Here's how the part is built. I have some questions about the finished solid (model axes, mm). A direction names the side the tool comes from. Round coordinates to 2 decimals unless told otherwise and drop trailing zeros. Write each loop counter-clockwise with the first axis right and the second up, starting at its lowest first coordinate (ties: lowest second). Pieces come first, ordered by that corner, then holes. Notation, with made-up numbers: (66, -31) -> (105, -31) arc R28 cw to (105, -13) -> close; hole circle Ø11 at (81.5, 58.5). An arc over 180 degrees is marked (long way). Put each result on its own line as item: value. Start each with the question number.
1) Which directions (+Z, -Z, +X, -X, +Y, -Y) give clear straight access to the entire face, cutting with the end or side of a thin tool? Please do faces 1 (the flat face through (7.4, 14, 9)), 2 (the flat face through (7, 21, 0)).
2) I want a section at A-A, the plane x = 0. List the corners of the cut face in (y, z) for me, then the cut area to 3 significant figures.
3) I want a section at C-C, the plane z = 0. List the corners of the cut face in (x, y) for me.
4) Will these pins go through, and if not, where does the flat tip stop? P1, Ø6, axis at x = 2, z = -4.5, coming from the +Y side; P2, Ø6, axis at x = 6, y = 15.5, coming from the +Z side; P3, Ø3, axis at y = 8, z = -6, coming from the -X side; P4, Ø5, axis at y = 10, z = 0, coming from the -X side.
5) We'd pull the mould along Z, two halves only. Please class faces 3 (the flat face through (7.4, 14, -9)), 4 (the flat face through (-2.4, 0, 1.9)), 5 (the cylindrical face through (8.521, 32.727, 0.358)): released by +Z, released by -Z, zero draft, split by the parting line, or undercut.
6) I want a section at D-D, the plane z = 7. List the corners of the cut face in (x, y) for me.
7) I want a section at B-B, the plane y = 10. List the corners of the cut face in (x, z) for me.
8) If I drill on line 1 along Y through (x, z) = (8.2, 0); line 2 along Z through (x, y) = (0, 0.8); line 3 along X through (y, z) = (22, 4.5), over which ranges is the centre line in solid material (lowest first)? Write a range as [from, to].
from build123d import *

# Parameters (mm, degrees)
SKETCH_1_W          = 20
SKETCH_1_H          = 18
EXTRUDE_1_DEPTH     = 3
SKETCH_2_W          = 3
SKETCH_2_H          = 18
EXTRUDE_2_DEPTH     = 37
SKETCH_4_R          = 2.75
CUT_EXTRUDE_1_DEPTH = 41
SKETCH_5_R          = 2.75
CUT_EXTRUDE_2_DEPTH = 21


with BuildPart() as part:
    # 草图1 → 凸台-拉伸1 (new body)
    with BuildSketch(Plane(origin=(0, 0, 0), x_dir=(1, 0, 0), z_dir=(0, 1, 0))):
        Rectangle(SKETCH_1_W, SKETCH_1_H)
    extrude(amount=EXTRUDE_1_DEPTH)

    # 草图2 → 凸台-拉伸2 (add)
    with BuildSketch(Plane(origin=(0, 3, 0), x_dir=(1, 0, 0), z_dir=(0, 1, 0))):
        with Locations((8.5, 0)):
            Rectangle(SKETCH_2_W, SKETCH_2_H)
    extrude(amount=EXTRUDE_2_DEPTH)

    # 草图4 → 切除-拉伸1 (cut, through all)
    with BuildSketch(Plane.XZ):
        Circle(SKETCH_4_R)
    extrude(amount=-CUT_EXTRUDE_1_DEPTH, mode=Mode.SUBTRACT)

    # 草图5 → 切除-拉伸2 (cut, through all)
    with BuildSketch(Plane(origin=(10, 0, 0), x_dir=(0, 0, -1), z_dir=(1, 0, 0))):
        with Locations((0, 10)):
            Circle(SKETCH_5_R)
        with Locations((0, 30)):
            Circle(SKETCH_5_R)
    extrude(amount=-CUT_EXTRUDE_2_DEPTH, mode=Mode.SUBTRACT)


solid = part.part
Findings:
1. face 1: +Z, +X, -X, +Y, -Y
1. face 2: +Z, -Z, -X, +Y
2. outline: (0, -9) -> (3, -9) -> (3, -2.75) -> (0, -2.75) -> close; (0, 2.75) -> (3, 2.75) -> (3, 9) -> (0, 9) -> close
2. area: 37.5 mm2
3. outline: (-10, 0) -> (-2.75, 0) -> (-2.75, 3) -> (-10, 3) -> close; (2.75, 0) -> (10, 0) -> (10, 7.25) -> (7, 7.25) -> (7, 3) -> (2.75, 3) -> close; (7, 12.75) -> (10, 12.75) -> (10, 27.25) -> (7, 27.25) -> close; (7, 32.75) -> (10, 32.75) -> (10, 40) -> (7, 40) -> close
4. P1: stops at y = 3
4. P2: stops at z = 9
4. P3: stops at x = 7
4. P4: passes through
5. face 3: released by -Z
5. face 4: zero draft
5. face 5: undercut
6. outline: (-10, 0) -> (10, 0) -> (10, 40) -> (7, 40) -> (7, 3) -> (-10, 3) -> close
7. outline: (7, -9) -> (10, -9) -> (10, -2.75) -> (7, -2.75) -> close; (7, 2.75) -> (10, 2.75) -> (10, 9) -> (7, 9) -> close
8. line 1: y = [0, 7.25], [12.75, 27.25], [32.75, 40]
8. line 2: z = [-9, -2.75], [2.75, 9]
8. line 3: x = [7, 10]
